Geometry check sheet. Reference: drawing and pictorial views, mm from the part's lowest x, y, z. Give positions to 0.01 mm unless a question says otherwise; leave off trailing zeros. Write each loop counter-clockwise with the first axis right and the second up, starting at its lowest first coordinate (ties: lowest second). Pieces come first, ordered by that corner, then holes. Notation, with made-up numbers: M -3.75,-25 L 37.25,-25 A23 ccw 37.25,-17 Z; hole C 9,78 d8. An arc over 180 degrees is marked long. One line per item, written item: value. Start each with the question number.
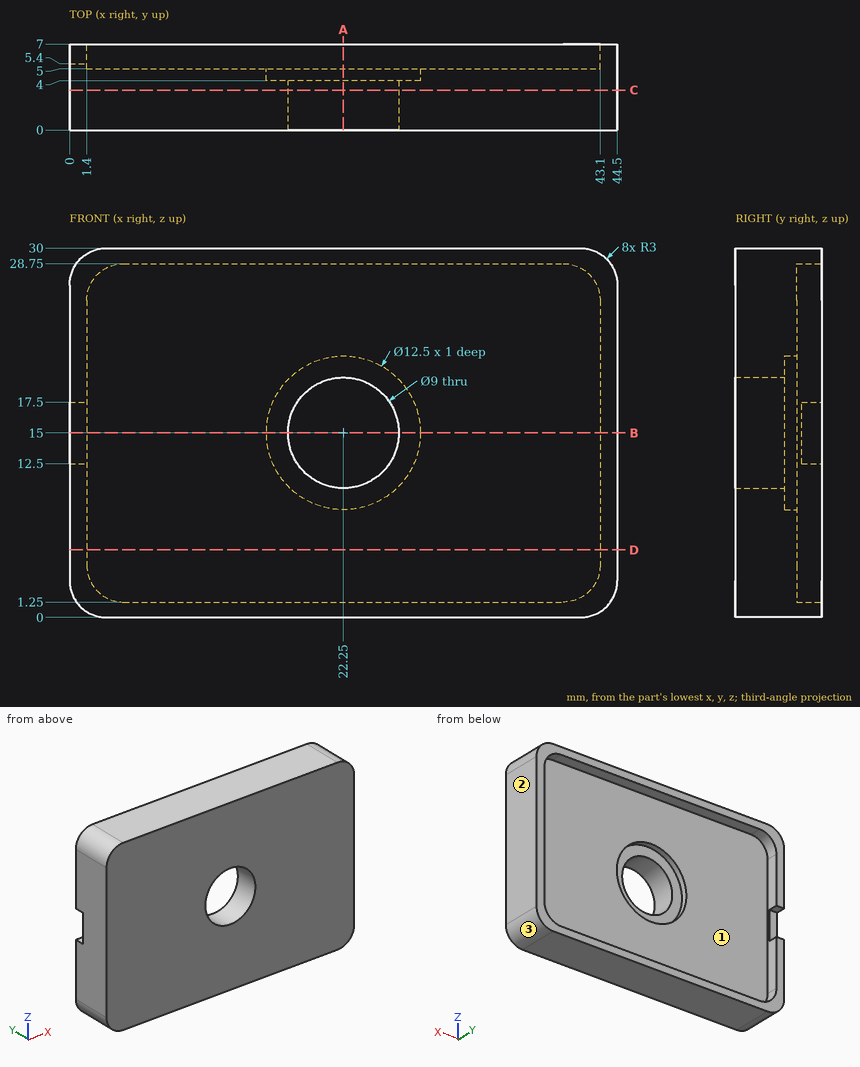
1) Cross-section at B-B (z = 15). Record the boundary of the cut face in (x, y).
2) Material ranges on L1, parallel to Z at x = 22.25, y = 1.3; L2, parallel to Z at x = 18, y = 6.5; L3, parallel to X at y = 5.25, z = 9, recorded low to high. Write a range as from..to.
3) Cross-section at D-D (z = 5.5). Record the boundary of the cut face in (x, y), plus the area to 3 significant figures.
4) Cross-section at A-A (x = 22.25). Record the boundary of the cut face in (y, z), plus the area to 4 significant figures.
5) Gauge pin test, flat ends, axial feed: pin 1 (4 mm diameter, centred on x = 6, z = 5.5, fed in from +Y); pin 2 (0.7 mm diameter, centred on x = 0.5, y = 6.5, fed in from +Z); pin 3 (7 mm diameter, centred on x = 22.25, z = 15, fed in from +Y). Record the tip position at first contact, or that the pin passes through.
6) Draft check along Z on the marked faces 1, 2 and 3. Enter one of: released by +Z, released by -Z, zero draft, split by the parting line, or undercut.
7) Cross-section at C-C (y = 3.25). Record the boundary of the cut face in (x, z).
Data:
1. outline: M 0,0 L 17.75,0 L 17.75,4 L 16,4 L 16,5 L 1.4,5 L 1.4,5.4 L 0,5.4 Z; M 26.75,0 L 44.5,0 L 44.5,7 L 43.1,7 L 43.1,5 L 28.5,5 L 28.5,4 L 26.75,4 Z
2. L1: z = 0..10.5, 19.5..30
2. L2: z = 0..1.25, 28.75..30
2. L3: x = 0..1.4, 43.1..44.5
3. outline: M 0,0 L 44.5,0 L 44.5,7 L 43.1,7 L 43.1,5 L 1.4,5 L 1.4,7 L 0,7 Z
3. area: 228 mm2
4. outline: M 0,0 L 7,0 L 7,1.25 L 5,1.25 L 5,8.75 L 4,8.75 L 4,10.5 L 0,10.5 Z; M 0,19.5 L 4,19.5 L 4,21.25 L 5,21.25 L 5,28.75 L 7,28.75 L 7,30 L 0,30 Z
4. area: 106.5 mm2
5. pin 1: stops at y = 5
5. pin 2: stops at z = 29.09
5. pin 3: passes through
6. face 1: undercut
6. face 2: zero draft
6. face 3: released by -Z
7. outline: M 0,3 A3 ccw 3,0 L 41.5,0 A3 ccw 44.5,3 L 44.5,27 A3 ccw 41.5,30 L 3,30 A3 ccw 0,27 Z; hole C 22.25,15 d9
